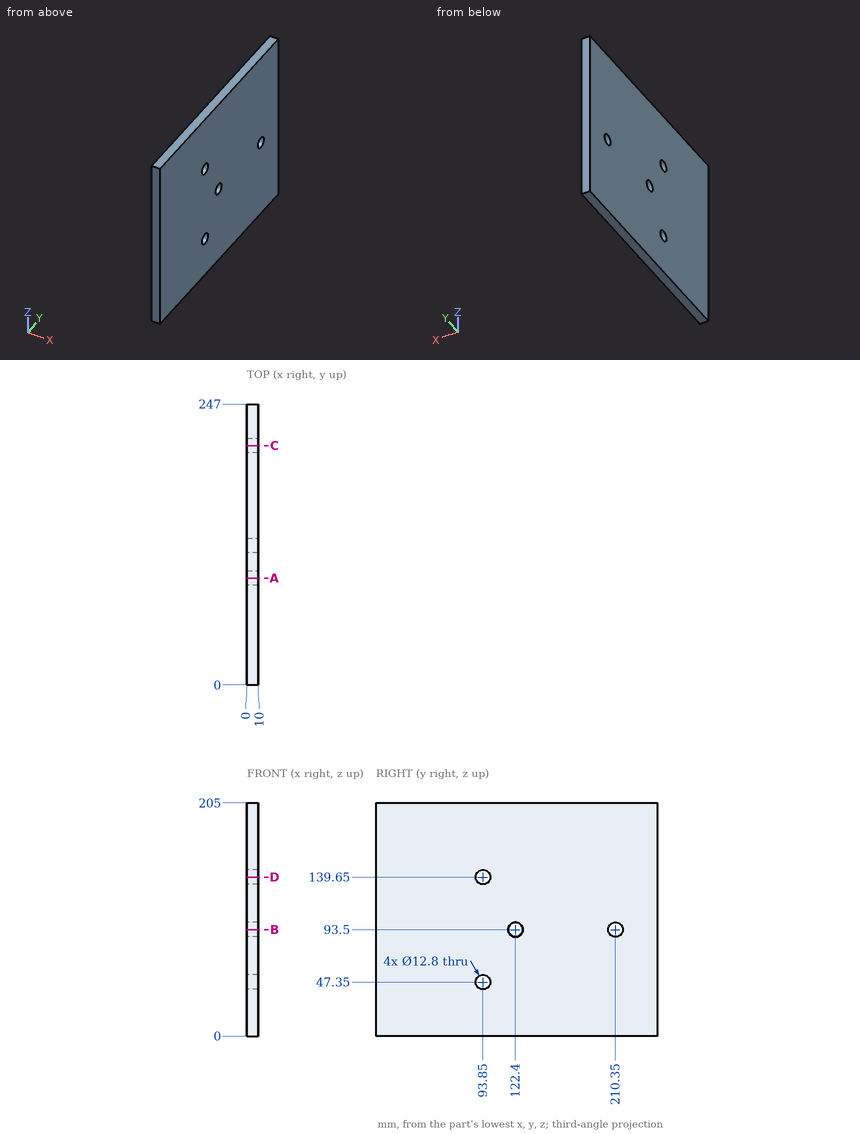
Drawing for the job (mm, zero at the part's lowest x, y, z). Coordinates: 2 decimals unless noted, no trailing zeros. Order: outer loops, then holes, each group sorted by start corner. A loop starts at its lowest first (then second) coordinate and runs counter-clockwise, first axis right, second up. Notation, with made-up numbers: (47, -28.75) -> (78, -28.75) arc R22 ccw to (78, 8.25) -> close; hole circle Ø5 at (45, 11.5). An arc over 180 degrees is marked (long way). One line per item, written item: value.
(1) Slice it at D-D, the plane z = 139.65. List the corners of the cut face in (x, y), plus the area to 3 significant figures.
Checked values:
outline: (0, 0) -> (10, 0) -> (10, 87.45) -> (0, 87.45) -> close; (0, 100.25) -> (10, 100.25) -> (10, 247) -> (0, 247) -> close
area: 2,340 mm2
(2) Drop a flat-ended pin along its axis: pin 1 Ø2 at (y, z) = (186, 86.5) entering from -X. Give the stop position or say it passes through.
Checked values:
pin 1: x = 0
(3) Slice it at B-B, the plane z = 93.5. List the corners of the cut face in (x, y), plus the area to 3 significant figures.
Checked values:
outline: (0, 0) -> (10, 0) -> (10, 116) -> (0, 116) -> close; (0, 128.8) -> (10, 128.8) -> (10, 203.95) -> (0, 203.95) -> close; (0, 216.75) -> (10, 216.75) -> (10, 247) -> (0, 247) -> close
area: 2,210 mm2
(4) Slice it at C-C, the plane y = 210.35. List the corners of the cut face in (x, z), plus the area to 3 significant figures.
Checked values:
outline: (0, 0) -> (10, 0) -> (10, 87.1) -> (0, 87.1) -> close; (0, 99.9) -> (10, 99.9) -> (10, 205) -> (0, 205) -> close
area: 1,920 mm2
(5) Probe line 1 (Z direction, x = 3.5, y = 93.85); line 2 (Z direction, x = 4.75, y = 210.35); line 3 (Z direction, x = 8.5, y = 117). List the from-to ranges inside material, lowest first. Write a range as [from, to].
Checked values:
line 1: [0, 40.95], [53.75, 133.25], [146.05, 205]
line 2: [0, 87.1], [99.9, 205]
line 3: [0, 90.06], [96.94, 205]
(6) Slice it at A-A, the plane y = 93.85. List the corners of the cut face in (x, z), plus the area to 3 significant figures.
Checked values:
outline: (0, 0) -> (10, 0) -> (10, 40.95) -> (0, 40.95) -> close; (0, 53.75) -> (10, 53.75) -> (10, 133.25) -> (0, 133.25) -> close; (0, 146.05) -> (10, 146.05) -> (10, 205) -> (0, 205) -> close
area: 1,790 mm2
